Source: CAD feature listing. Evaluate the final solid. Frame: model axes, mm. Coordinates: 2 decimals unless noted, no trailing zeros. Write each loop counter-clockwise with the first axis right and the second up, starting at its lowest first coordinate (ties: lowest second). Pieces come first, ordered by that corner, then holes. Notation, with made-up numbers: M 72,-28.75 L 118,-28.75 A26 cw 118,0.25 Z; hole C 51.25,15.25 d6. An arc over 180 degrees is marked long. One line per item, written item: value. Start each with the question number.
Item 1: Pin query (flat end, axial travel): P1, Ø1.5, axis at x = 7.5, y = 4.15, coming from the -Z side (3 decimals); P2, Ø3, axis at x = -7.5, y = 4.15, coming from the -Z side. Return the tip coordinate at first contact, or that it passes through.
Item 2: Mould query, pull axis X, two halves, no side actions, for faces 1 (the cylindrical face through (0.324, 4.092, 2.696)), 2 (the cylindrical face through (-0.3, 4.1, 0.7)), 3 (the flat face through (22.5, 4, 0)). Classes: released by +X, released by -X, zero draft, split by the parting line, or undercut.
Item 3: Ray query, L1, parallel to X at y = 4.15, z = 1; L2, parallel to Y at x = 7.5, z = 1.3; L3, parallel to Z at x = -1, y = 2.5. Return the intervals inside material, ascending. Write a range as from..to.
Item 4: Cut plane B-B, the plane y = 4.15. Output: boundary loops of the cut face in (x, z).
Item 5: Cut plane D-D, the plane y = 7.5. Output: boundary loops of the cut face in (x, z).
Item 6: Cut plane A-A, the plane x = -7.5. Output: boundary loops of the cut face in (y, z).
```python
from build123d import *

# Parameters (mm, degrees)
BOSS_EXTRUDE1_DEPTH     = 8.3
SKETCH2_R               = 1.25
CUT_EXTRUDE1_DEPTH      = 3.700074126
CUT_EXTRUDE1_DEPTH_BACK = 1.960467608


with BuildPart() as part:
    # Sketch1 → Boss-Extrude1 (new body)
    with BuildSketch(Plane(origin=(0, 0, 0), x_dir=(1, 0, 0), z_dir=(0, 1, 0))):
        with BuildLine():
            Line((22.5, 0.960467608), (22.5, -1.059592066))
            ThreePointArc((22.5, -1.059592066), (0.00793889, -2.697795715), (-22.5, -1.2945099))
            Line((-22.5, -1.2945099), (-22.5, 0.722652417))
            ThreePointArc((-22.5, 0.722652417), (0.008135008, -0.697767096), (22.5, 0.960467608))
        make_face()
    extrude(amount=BOSS_EXTRUDE1_DEPTH)

    # Sketch2 → Cut-Extrude1 (cut, two sides)
    with BuildSketch(Plane.XY) as cut_extrude1_sk:
        with Locations((7.5, 4.15)):
            Circle(SKETCH2_R)
        with Locations((-7.5, 4.15)):
            Circle(SKETCH2_R)
    extrude(amount=CUT_EXTRUDE1_DEPTH, mode=Mode.SUBTRACT)
    extrude(cut_extrude1_sk.sketch, amount=-CUT_EXTRUDE1_DEPTH_BACK, mode=Mode.SUBTRACT)


solid = part.part
```
From the geometry:
1. P1: passes through
1. P2: stops at z = 0.5
2. face 1: split by the parting line
2. face 2: undercut
2. face 3: released by +X
3. L1: x = -22.5..-8.75, -6.25..6.25, 8.75..22.5
3. L2: y = 0..2.9, 5.4..8.3
3. L3: z = 0.7..2.7
4. outline: M -22.5,-0.72 A165.21 cw -8.75,0.51 L -8.75,2.51 A167.21 ccw -22.5,1.29 Z; M -6.25,0.61 A165.21 cw 6.25,0.55 L 6.25,2.55 A167.21 ccw -6.25,2.61 Z; M 8.75,0.42 A165.21 cw 22.5,-0.96 L 22.5,1.06 A167.21 ccw 8.75,2.42 Z
5. outline: M -22.5,-0.72 A165.21 cw 22.5,-0.96 L 22.5,1.06 A167.21 ccw -22.5,1.29 Z
6. outline: M 0,0.57 L 2.9,0.57 L 2.9,2.57 L 0,2.57 Z; M 5.4,0.57 L 8.3,0.57 L 8.3,2.57 L 5.4,2.57 Z
